Solid Edge part; units mm, degrees
sketch "Sketch1" plane through (0, 0, 0) normal (0, 0, 1) x (1, 0, 0)
  circle A0 centre (0, 0) radius 25
extrude "Protrusion1" add sketch "Sketch1" against normal blind 3.1
sketch "Sketch2" plane through (0, 0, -3.1) normal (0, 0, -1) x (1, 0, 0)
  circle A0 centre (0, 0) radius 20.5
extrude "Protrusion2" add sketch "Sketch2" along normal blind 3.2
hole "Hole1" at (0, 0, 0) direction (0, 0, -1) diameter 19 end up to next
chamfer "Chamfer1" distance 0.5 angle 45 2 edges at (-9.5, 0, -6.3) (-9.5, 0, 0)
properties part number "75356"
The listing builds one solid part. Answer for the finished solid, in the listing's coordinates (mm). A direction names the side the tool comes from. Give positions to 0.01 mm unless a question says otherwise; leave off trailing zeros. Loops run counter-clockwise (first coordinate to the right, second up) from the corner with the lowest first, then second, coordinate; pieces in that order, holes last. Notation, with made-up numbers: M 15,-19 L 61,-19 A21 cw 61,16 Z; hole C -17.5,21 d10. An arc over 180 degrees is marked long. Answer as CSV lines item,"result".
Item 1: The mould has two halves that part along Y. Classify faces 1 (the flat face through (0, -11, 0)), 2 (the cylindrical face through (-8.43, -4.38, -3.11)), 3 (the cylindrical face through (-4.444, -20.013, -4.678)): released by +Y, released by -Y, zero draft, split by the parting line, or undercut.
Values follow:
face 1,"zero draft"
face 2,"undercut"
face 3,"split by the parting line"
Item 2: Which of the six approach directions +Z, -Z, +X, -X, +Y, -Y give full straight-line access (tool end or side, diameter ignored) to faces 4 (the flat face through (-3.8, 20.5, -3.1)), 5 (the cylindrical face through (23.846, 7.509, -1.528))?
Values follow:
face 4,"-Z"
face 5,"+Z, -Z"
Item 3: Given pin 1 Ø2 at (y, z) = (-12.5, -1) entering from -X; pin 2 Ø2 at (x, z) = (19.5, -1.5) entering from -Y; pin 3 Ø3 at (y, z) = (-15.5, -0.5) entering from +X, each flat-ended and moving along its own axis, determine where each tip first touches the part or whether it passes through.
Values follow:
pin 1,"stops at x = -22.2"
pin 2,"stops at y = -16.82"
pin 3,"stops at x = 20.71"
Item 4: Straight lines are drawn through the part: line 1 along X through (y, z) = (0, -3.2); line 2 along Y through (x, z) = (0, -1.9); line 3 along Z through (x, y) = (21.5, 9). For each, find the intervals that lie inside material, in ascending order. Write a range as [from, to].
Values follow:
line 1,"x = [-20.5, -9.5], [9.5, 20.5]"
line 2,"y = [-25, -9.5], [9.5, 25]"
line 3,"z = [-3.1, 0]"
Item 5: The part is cut by section D-D (y = 16). Give the vertices of the cut face in (x, z).
Values follow:
outline,"M -19.21,-3.1 L -12.82,-3.1 L -12.82,-6.3 L 12.82,-6.3 L 12.82,-3.1 L 19.21,-3.1 L 19.21,0 L -19.21,0 Z"
Item 6: The part is cut by section A-A (y = 0). Give the vertices of the cut face in (x, z).
Values follow:
outline,"M -25,-3.1 L -20.5,-3.1 L -20.5,-6.3 L -10,-6.3 L -9.5,-5.8 L -9.5,-0.5 L -10,0 L -25,0 Z; M 9.5,-5.8 L 10,-6.3 L 20.5,-6.3 L 20.5,-3.1 L 25,-3.1 L 25,0 L 10,0 L 9.5,-0.5 Z"
Item 7: The part is cut by section C-C (z = -2.25). Give the vertices of the cut face in (x, y), and give its area (3 significant figures).
Values follow:
outline,"C 0,0 d50; hole C 0,0 d19"
area,"1,680 mm^2"
